The listing builds one solid part. Answer for the finished solid, in the listing's coordinates (mm). Coordinates: 2 decimals unless noted, no trailing zeros. Write each loop counter-clockwise with the first axis right and the second up, starting at its lowest first coordinate (ties: lowest second). Pieces come first, ordered by that corner, then holes. Notation, with made-up numbers: M 9.5,65 L 47.5,65 A9 ccw 47.5,72 Z; hole C -13.75,83.5 d2. An arc over 180 degrees is marked long. Put each result on its own line as item: value. Start each with the question number.
```python
from build123d import *

# Parameters (mm, degrees)
SKETCH1_R           = 1.5
BOSS_EXTRUDE1_DEPTH = 1.61
SKETCH2_W           = 12
SKETCH2_H           = 3.22
CUT_EXTRUDE1_DEPTH  = 3.22
LPATTERN1_COUNT     = 9
LPATTERN1_PITCH     = 24


with BuildPart() as part:
    # Sketch1 → Boss-Extrude1 (new body, symmetric)
    with BuildSketch(Plane.XY):
        Polygon((-95.775442885, -4.703941319), (-115.775442885, 5.296058681), (107.831354865, 5.296058681), (102.831354865, -4.703941319), align=None)
        Circle(SKETCH1_R, mode=Mode.SUBTRACT)
    extrude(amount=BOSS_EXTRUDE1_DEPTH, both=True)

    # Sketch2 → Cut-Extrude1 (cut)
    with BuildSketch(Plane.XY.offset(1.61)):
        with Locations((-97.775442885, 3.686058681)):
            Rectangle(SKETCH2_W, SKETCH2_H)
    cut_extrude1 = extrude(amount=-CUT_EXTRUDE1_DEPTH, mode=Mode.SUBTRACT)

    # LPattern1: Cut-Extrude1 ×9
    with Locations(*[(i * LPATTERN1_PITCH, 0, 0) for i in range(1, LPATTERN1_COUNT)]):
        add(cut_extrude1, mode=Mode.SUBTRACT)


solid = part.part
```
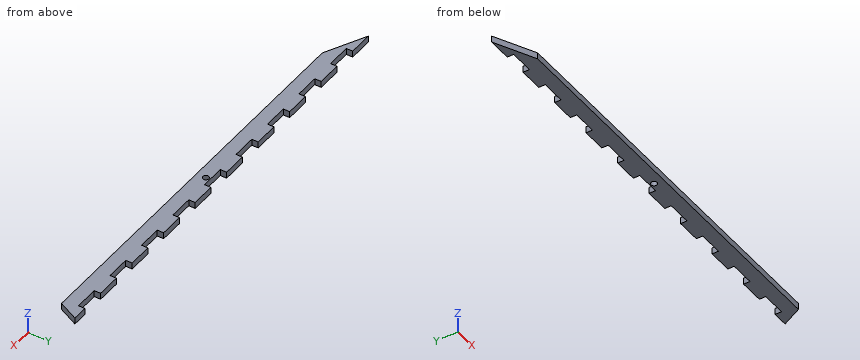
1) A cutting plane is placed at A-A on x = -49. Write down the section's boundary in (y, z).
2) Straight lines are drawn through the part: probe 1 along Y at (x, z) = (0, -0.35); probe 2 along Y at (x, z) = (-68, -1.1); probe 3 along X at (y, z) = (1, -1.1). For each, find the intervals that lie inside material, in ascending order.
3) Given pin 1 Ø1.6 at (y, z) = (3, -0.5) entering from -X; pin 2 Ø5 at (x, y) = (0, 0) entering from +Z; pin 3 Ø1 at (x, z) = (23, 0.5) entering from +Y; pin 4 Ø1 at (y, z) = (3.5, -0.5) entering from +X, each flat-ended and moving along its own axis, determine where each tip first touches the part or whether it passes through.
Answers follow:
1. outline: M -4.7,-1.61 L 2.08,-1.61 L 2.08,1.61 L -4.7,1.61 Z
2. probe 1: y = -4.7 to -1.5, 1.5 to 2.08
2. probe 2: y = -4.7 to 2.08
2. probe 3: x = -107.18 to -1.12, 1.12 to 105.68
3. pin 1: stops at x = -112.78
3. pin 2: stops at z = 1.61
3. pin 3: stops at y = 2.08
3. pin 4: stops at x = 107.18
